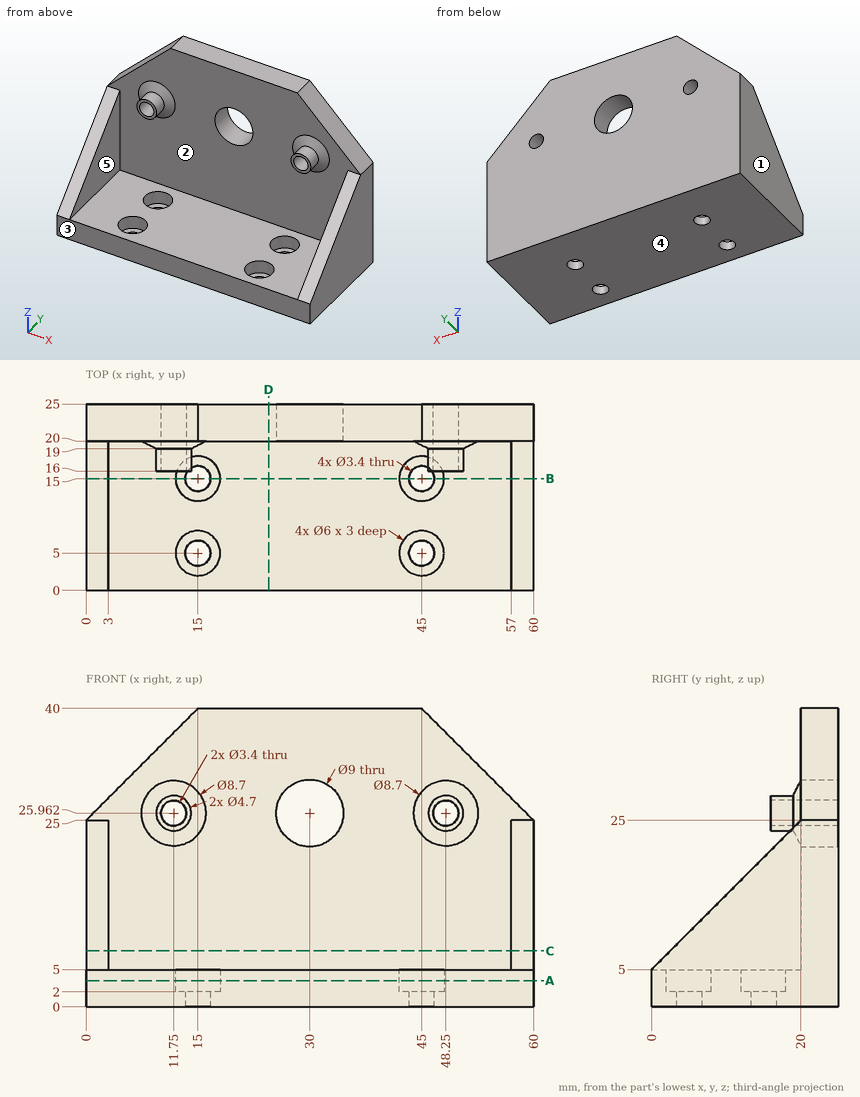
Study the drawing (mm; zero at the part's minimum x, y, z) and answer. A direction names the side the tool comes from. Coordinates: 2 decimals unless noted, no trailing zeros. Write each loop counter-clockwise with the first axis right and the second up, starting at its lowest first coordinate (ties: lowest second). Pieces come first, ordered by that corner, then holes. Notation, with made-up numbers: (71.5, 1) - (118.5, 1) arc R5 cw to (118.5, 10) - close; hole circle Ø2 at (-17, 40.25). An arc over 180 degrees is marked (long way). Put each result on its own line as item: value.
1. Flat-ended cylindrical pins translate along their axes: pin 1 Ø3.5 at (x, y) = (15, 5) entering from +Z; pin 2 Ø1.5 at (x, z) = (13, 26.5) entering from -Y; pin 3 Ø5 at (x, z) = (13, 10.5) entering from -Y. Find the tip coordinate at first contact, or state that the pin passes through.
Answer sheet:
pin 1: stops at z = 2
pin 2: stops at y = 16
pin 3: stops at y = 20
2. Determine the mould class of the marked faces 1, 2 and 3 for opening direction X: pulls with the +X half, pulls with the -X half, needs draft (parallel to the pull), parting line crosses it, or undercut.
Answer sheet:
face 1: pulls with the -X half
face 2: undercut
face 3: needs draft
3. The part is cut by section B-B on y = 15. Give the vertices of the cut face in (x, z).
Answer sheet:
outline: (0, 0) - (13.3, 0) - (13.3, 2) - (12, 2) - (12, 5) - (3, 5) - (3, 20) - (0, 20) - close; (16.7, 0) - (43.3, 0) - (43.3, 2) - (42, 2) - (42, 5) - (18, 5) - (18, 2) - (16.7, 2) - close; (46.7, 0) - (60, 0) - (60, 20) - (57, 20) - (57, 5) - (48, 5) - (48, 2) - (46.7, 2) - close
4. The part is cut by section C-C on z = 7.5. Give the vertices of the cut face in (x, y).
Answer sheet:
outline: (0, 2.5) - (3, 2.5) - (3, 20) - (57, 20) - (57, 2.5) - (60, 2.5) - (60, 25) - (0, 25) - close
5. The part is cut by section A-A on z = 3.5. Give the vertices of the cut face in (x, y), plus the area to 3 significant figures.
Answer sheet:
outline: (0, 0) - (60, 0) - (60, 25) - (0, 25) - close; hole circle Ø6 at (15, 5); hole circle Ø6 at (15, 15); hole circle Ø6 at (45, 5); hole circle Ø6 at (45, 15)
area: 1,390 mm^2
6. A tool of negligible diameter and unlimited length cuts with its end or side. For the marked faces 4 and 5, from which of +Z, -Z, +X, -X, +Y, -Y can it reach the whole face along a straight path? Write none if from no direction.
Answer sheet:
face 4: -Z, +X, -X, +Y, -Y
face 5: +Z, -Y
7. The part is cut by section D-D on x = 24.5. Give the vertices of the cut face in (y, z).
Answer sheet:
outline: (0, 0) - (25, 0) - (25, 40) - (20, 40) - (20, 5) - (0, 5) - close
8. Find the intervals of material crossed by line 1 along X through (y, z) = (5, 1.1); line 2 along Y through (x, z) = (45, 0.65); line 3 along Y through (x, z) = (15, 3.8), in increasing order. Write a range as from..to.
Answer sheet:
line 1: x = 0..13.3, 16.7..43.3, 46.7..60
line 2: y = 0..3.3, 6.7..13.3, 16.7..25
line 3: y = 0..2, 8..12, 18..25
